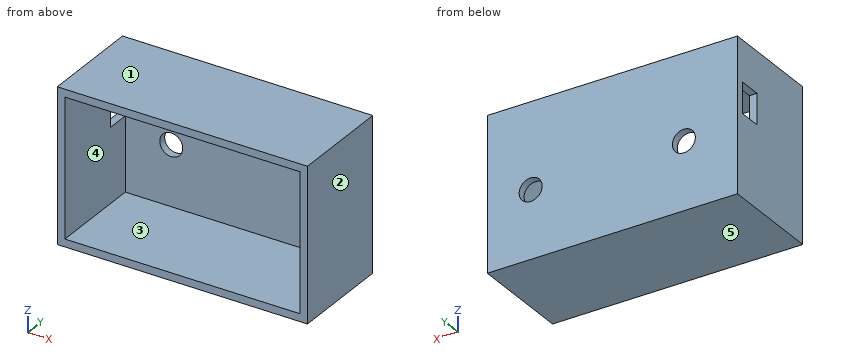
```python
from build123d import *

# Parameters (mm, degrees)
F0_W     = 49
F0_H     = 30
F1_DEPTH = 20
F2_T     = -1.5
F3_R     = 2.25
F4_DEPTH = 1.5
F5_W     = 4.5
F5_H     = 6
F6_DEPTH = 1.5


with BuildPart() as f1:
    # F0 (on Front) → F1 (new body)
    with BuildSketch(Plane.XZ):
        with Locations((1.226867, 1.730894)):
            Rectangle(F0_W, F0_H)
    extrude(amount=F1_DEPTH)

    # F2
    f2_openings = [f1.faces().sort_by_distance(p)[0] for p in [
        (1.226867, -20, 1.730894),
    ]]
    offset(amount=F2_T, openings=f2_openings)

    # F3 (on face) → F4 (cut, through all)
    with BuildSketch(Plane.XZ.offset(1.5)):
        with Locations((-12.773133, 0)):
            Circle(F3_R)
        with Locations((17.226867, 0)):
            Circle(F3_R)
    extrude(amount=-F4_DEPTH, mode=Mode.SUBTRACT)

    # F5 (on face) → F6 (cut, through all)
    with BuildSketch(Plane(origin=(-23.273133, 0, 0), x_dir=(0, -1, 0), z_dir=(-1, 0, 0))):
        with Locations((3.75, 5.730894)):
            Rectangle(F5_W, F5_H)
    extrude(amount=-F6_DEPTH, mode=Mode.SUBTRACT)


solid = f1.part
```
Build history of the part. All positions in model axes, mm. Face numbers are marked on the shaded views. A direction names the side the tool comes from. Round coordinates to 2 decimals unless told otherwise and drop trailing zeros. Write each loop counter-clockwise with the first axis right and the second up, starting at its lowest first coordinate (ties: lowest second). Pieces come first, ordered by that corner, then holes.
1) Pin check, flat tips, straight feed: pin 1 (1.2 mm diameter, centred on x = -22.5, z = 7, fed in from +Y); pin 2 (3.5 mm diameter, centred on x = -12.77, z = 0, fed in from -Y); pin 3 (1.5 mm diameter, centred on x = 18, z = -2, fed in from -Y). Stop position of each tip, or through.
2) Band-saw the part on B-B, the plane y = -11.5. List the corners of the cut face in (x, z), and give its area (3 significant figures).
3) Mould opens along X. For the marked faces 1, 2 and 3 say: +X half, -X half, draft (parallel to the pull), parting line (faces both ways), or undercut.
4) Band-saw the part on A-A, the plane z = 0. List the corners of the cut face in (x, y).
5) Band-saw the part on C-C, the plane z = 6.75. List the corners of the cut face in (x, y), and give its area (3 significant figures).
6) 3-axis set-ups, long thin cutter, end or side, ignore diameter. For the marked faces 4 and 5: which of +Z, -Z, +X, -X, +Y, -Y reach the whole face in a straight line?
7) Drill centre lines: probe 1 along Z at (x, y) = (10, -16.25); probe 2 along X at (y, z) = (-13.25, -6.5); probe 3 along Y at (x, z) = (18, -6.5). Where is each one in solid material? Low to high.
8) Band-saw the part on D-D, the plane x = 0. List the corners of the cut face in (y, z).
Ans:
1. pin 1: stops at y = 0
1. pin 2: passes through
1. pin 3: stops at y = -1.5
2. outline: (-23.27, -13.27) - (25.73, -13.27) - (25.73, 16.73) - (-23.27, 16.73) - close; hole (-21.77, -11.77) - (24.23, -11.77) - (24.23, 15.23) - (-21.77, 15.23) - close
2. area: 228 mm2
3. face 1: draft
3. face 2: +X half
3. face 3: undercut
4. outline: (-23.27, -20) - (-21.77, -20) - (-21.77, -1.5) - (-15.02, -1.5) - (-15.02, 0) - (-23.27, 0) - close; (-10.52, -1.5) - (14.98, -1.5) - (14.98, 0) - (-10.52, 0) - close; (19.48, -1.5) - (24.23, -1.5) - (24.23, -20) - (25.73, -20) - (25.73, 0) - (19.48, 0) - close
5. outline: (-23.27, -20) - (-21.77, -20) - (-21.77, -6) - (-23.27, -6) - close; (-23.27, -1.5) - (24.23, -1.5) - (24.23, -20) - (25.73, -20) - (25.73, 0) - (-23.27, 0) - close
5. area: 122 mm2
6. face 4: -Y
6. face 5: -Z, +X, -X, +Y, -Y
7. probe 1: z = -13.27 to -11.77, 15.23 to 16.73
7. probe 2: x = -23.27 to -21.77, 24.23 to 25.73
7. probe 3: y = -1.5 to 0
8. outline: (-20, -13.27) - (0, -13.27) - (0, 16.73) - (-20, 16.73) - (-20, 15.23) - (-1.5, 15.23) - (-1.5, -11.77) - (-20, -11.77) - close
